The drawing under review shows one solid part. Ordinate dimensions are in mm from its lowest x, y, z. Coordinates: 2 decimals unless noted, no trailing zeros. Loops run counter-clockwise (first coordinate to the right, second up) from the corner with the lowest first, then second, coordinate; pieces in that order, holes last. Notation, with made-up numbers: (75.25, 30) - (114.25, 30) arc R21 ccw to (114.25, 40) - close; hole circle Ø8 at (5, -37). An arc over 180 degrees is marked (long way). Use one line per item in the form item = value. Start each with the question number.
1. Add section A-A on x = 50.8. Give the boundary of the cut face in (y, z) (1 decimal).
2. To check wall thickness, follow probe 1 along Z at (x, y) = (50.8, 1.7); probe 2 along X at (y, z) = (1.1, 27.5); probe 3 along Z at (x, y) = (52, 2.65) (1 decimal). State the ranges of each line that lie inside material, in increasing order.
3. Add section D-D on z = 37.5. Give the boundary of the cut face in (x, y) (1 decimal).
4. For pin 1 Ø1 at (y, z) = (2.5, 84.5) entering from -X; pin 2 Ø1.5 at (y, z) = (2, 22) entering from +X; pin 3 Ø1.5 at (x, y) = (10, 0.5) entering from -Z, all flat-tipped, find the tip position at first contact; note any pin that passes through.
5. Add section B-B on y = 1.65. Give the boundary of the cut face in (x, z) (1 decimal).
6. Add section C-C on z = 73.5. Give the boundary of the cut face in (x, y) (1 decimal).
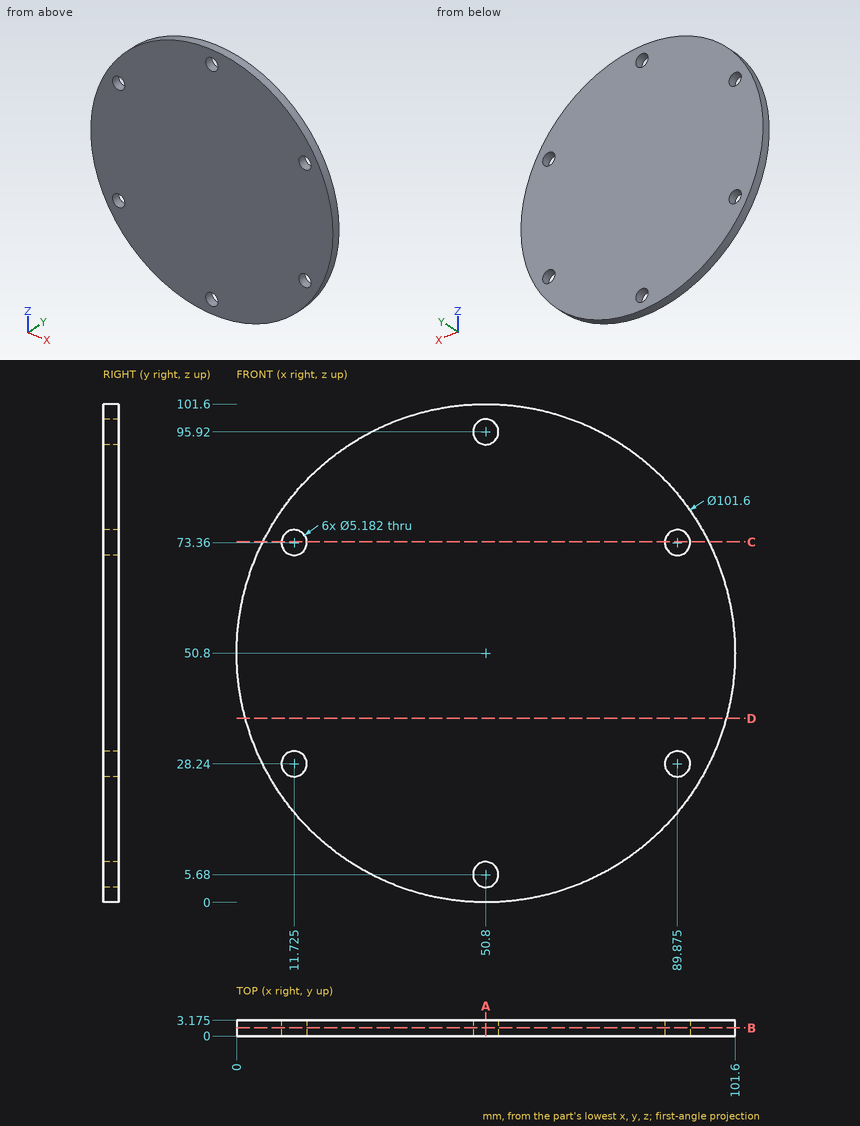
Conclusion:
q1.outline = (0, 0) - (3.2, 0) - (3.2, 3.1) - (0, 3.1) - close; (0, 8.3) - (3.2, 8.3) - (3.2, 93.3) - (0, 93.3) - close; (0, 98.5) - (3.2, 98.5) - (3.2, 101.6) - (0, 101.6) - close
q2.probe_1 = 0 to 3.09, 8.27 to 93.33, 98.51 to 101.6
q2.probe_2 = 5.66 to 9.24, 14.21 to 87.39, 92.36 to 95.94
q2.probe_3 = 0 to 3.4, 8 to 93.6, 98.2 to 101.6
q3.outline = (1.8, 0) - (99.8, 0) - (99.8, 3.2) - (1.8, 3.2) - close
q4.pin_1 = 12.35
q4.pin_2 = 93.15
q4.pin_3 = 19.55
q5.outline = circle Ø101.6 at (50.8, 50.8); hole circle Ø5.2 at (11.7, 28.2); hole circle Ø5.2 at (11.7, 73.4); hole circle Ø5.2 at (50.8, 5.7); hole circle Ø5.2 at (50.8, 95.9); hole circle Ø5.2 at (89.9, 28.2); hole circle Ø5.2 at (89.9, 73.4)
q6.outline = (5.4, 0) - (9.1, 0) - (9.1, 3.2) - (5.4, 3.2) - close; (14.3, 0) - (87.3, 0) - (87.3, 3.2) - (14.3, 3.2) - close; (92.5, 0) - (96.2, 0) - (96.2, 3.2) - (92.5, 3.2) - close
